Build history of the part. All positions in model axes, mm. A direction names the side the tool comes from. Round coordinates to 2 decimals unless told otherwise and drop trailing zeros. Loops run counter-clockwise (first coordinate to the right, second up) from the corner with the lowest first, then second, coordinate; pieces in that order, holes last.
from build123d import *

# Parameters (mm, degrees)
ESQUISSE1_W             = 240
ESQUISSE1_H             = 150
BOSS_EXTRU_1_DEPTH      = 40
ENL_V_MAT_EXTRU_1_DEPTH = 20
ESQUISSE2_3_R           = 15
ENL_V_MAT_EXTRU_2_DEPTH = 10
ESQUISSE2_4_R           = 22.5
ENL_V_MAT_EXTRU_3_DEPTH = 148.054411699
ESQUISSE2_5_R           = 22.5
ENL_V_MAT_EXTRU_4_DEPTH = 20


with BuildPart() as part:
    # Esquisse1 → Boss.-Extru.1 (new body)
    with BuildSketch(Plane.XY):
        Rectangle(ESQUISSE1_W, ESQUISSE1_H)
    extrude(amount=BOSS_EXTRU_1_DEPTH)

    # Esquisse2 → Enl_v. mat.-Extru.1 (cut)
    with BuildSketch(Plane.XY.offset(40)):
        with BuildLine():
            Line((-105, -30), (-105, 40))
            ThreePointArc((-105, 40), (-85, 60), (-65, 40))
            Line((-65, 40), (-65, -30))
            ThreePointArc((-65, -30), (-85, -50), (-105, -30))
        make_face()
    extrude(amount=-ENL_V_MAT_EXTRU_1_DEPTH, mode=Mode.SUBTRACT)

    # Esquisse2_3 → Enl_v. mat.-Extru.2 (cut)
    with BuildSketch(Plane.XY.offset(40)):
        with Locations((10, 45)):
            Circle(ESQUISSE2_3_R)
        with Locations((80, 45)):
            Circle(ESQUISSE2_3_R)
    extrude(amount=-ENL_V_MAT_EXTRU_2_DEPTH, mode=Mode.SUBTRACT)

    # Esquisse2_4 → Enl_v. mat.-Extru.3 (cut, through all)
    with BuildSketch(Plane.XY.offset(40)):
        with Locations((15, -30)):
            Circle(ESQUISSE2_4_R)
    extrude(amount=-ENL_V_MAT_EXTRU_3_DEPTH, mode=Mode.SUBTRACT)

    # Esquisse2_5 → Enl_v. mat.-Extru.4 (cut)
    with BuildSketch(Plane.XY.offset(40)):
        with BuildLine():
            Line((120, -75), (120, 15))
            Line((120, 15), (15, 15))
            ThreePointArc((15, 15), (-16.819805153, 1.819805153), (-30, -30))
            Line((-30, -30), (-30, -75))
            Line((-30, -75), (120, -75))
        make_face()
        with Locations((15, -30)):
            Circle(ESQUISSE2_5_R, mode=Mode.SUBTRACT)
    extrude(amount=-ENL_V_MAT_EXTRU_4_DEPTH, mode=Mode.SUBTRACT)


solid = part.part
(1) Probe line 1 (Y direction, x = 15, z = 9); line 2 (Y direction, x = 80, z = 37.75); line 3 (X direction, y = 56, z = 33). List the from-to ranges inside material, lowest first.
Responses:
line 1: y = -75 to -52.5, -7.5 to 75
line 2: y = 15 to 30, 60 to 75
line 3: x = -120 to -97, -73 to -0.2, 20.2 to 69.8, 90.2 to 120
(2) Which spindle directions (+Z, -Z, +X, -X, +Y, -Y) get a long thin tool onto all of the face, cutting with end or side? Do faces 1 (the face through (-85, -50, 30)), 2 (the face through (-28, 18, 40)), 3 (the face through (68, 15, 30)). Say none if no direction does.
Responses:
face 1: +Z
face 2: +Z, +X, -X, +Y, -Y
face 3: +Z, +X, -Y
(3) Slice it at C-C on x = 10. List the corners of the cut face in (y, z), plus the area to 3 significant figures.
Responses:
outline: (-75, 0) - (-51.94, 0) - (-51.94, 20) - (-75, 20) - close; (-8.06, 0) - (75, 0) - (75, 40) - (60, 40) - (60, 30) - (30, 30) - (30, 40) - (14.72, 40) - (14.72, 20) - (-8.06, 20) - close
area: 3,030 mm2
(4) Slice it at B-B on z = 36. List the corners of the cut face in (x, y).
Responses:
outline: (-120, -75) - (-30, -75) - (-30, -30) arc R45 cw to (15, 15) - (120, 15) - (120, 75) - (-120, 75) - close; hole (-105, -30) arc R20 ccw to (-65, -30) - (-65, 40) arc R20 ccw to (-105, 40) - close; hole circle Ø30 at (10, 45); hole circle Ø30 at (80, 45)
(5) Pull direction Y, two halves, no side cores. Call faces 4 (the face through (80, 45, 30)), 5 (the face through (-16.468, 2.168, 30.14)), 6 (the face through (8.047, 59.872, 35.07)), 7 (the face through (120, 16, 15)): +Y half, -Y half, draft (parallel to the pull), parting line (faces both ways), or undercut.
Responses:
face 4: undercut
face 5: -Y half
face 6: undercut
face 7: draft
(6) Slice it at A-A on y = -41.5. List the corners of the cut face in (x, z), plus the area to 3 significant figures.
Responses:
outline: (-120, 0) - (-4.34, 0) - (-4.34, 20) - (-30, 20) - (-30, 40) - (-68.64, 40) - (-68.64, 20) - (-101.36, 20) - (-101.36, 40) - (-120, 40) - close; (34.34, 0) - (120, 0) - (120, 20) - (34.34, 20) - close
area: 5,170 mm2
(7) Slice it at D-D on z = 3.5. List the corners of the cut face in (x, y).
Responses:
outline: (-120, -75) - (120, -75) - (120, 75) - (-120, 75) - close; hole circle Ø45 at (15, -30)
(8) Pin check, flat tips, straight feed: P1, Ø10, axis at x = 20.5, z = 32, coming from the -Y side; P2, Ø20, axis at x = -88.5, y = 24, coming from the +Z side; P3, Ø16, axis at y = -54, z = 30, coming from the +X side. Stop position of each tip, or through.
Responses:
P1: stops at y = 15
P2: stops at z = 20
P3: stops at x = -30
